```python
from build123d import *

# Parameters (mm, degrees)
CROQUIS4_R                = 1.5
SALIENTE_EXTRUIR1_DEPTH   = 5
SALIENTE_EXTRUIR1_2_DEPTH = 5
SALIENTE_EXTRUIR1_3_DEPTH = 5
SALIENTE_EXTRUIR2_START   = -3
CROQUIS5_R                = 1.5
SALIENTE_EXTRUIR2_DEPTH   = 3


with BuildPart() as part:
    # Croquis4 → Saliente-Extruir1 (new body)
    with BuildSketch(Plane.XY):
        with BuildLine():
            Line((31.332082611, 76.5), (31.332082611, 73.5))
            ThreePointArc((31.332082611, 73.5), (17.593960897, 62.317888205), (18.123970441, 44.612106598))
            Line((18.123970441, 44.612106598), (33.120139436, 16.408414688))
            ThreePointArc((33.120139436, 16.408414688), (31.879711346, 12.351157221), (27.822453879, 13.591585312))
            Line((27.822453879, 13.591585312), (17.849832742, 32.347357814))
            ThreePointArc((17.849832742, 32.347357814), (16.010285152, 34.285836504), (13.435094777, 35))
            Line((13.435094777, 35), (8.180668456, 35))
            ThreePointArc((8.180668456, 35), (4.835015424, 33.715724127), (3.208058979, 30.522642316))
            Line((3.208058979, 30.522642316), (1.105974274, 10.522642316))
            Line((1.105974274, 10.522642316), (-1.894025726, 10.522642316))
            Line((-1.894025726, 10.522642316), (-1.894025726, 27.20144431))
            ThreePointArc((-1.894025726, 27.20144431), (-0.837875871, 33.61475404), (2.219028442, 39.350722155))
            ThreePointArc((2.219028442, 39.350722155), (5.275932756, 45.086690271), (6.332082611, 51.5))
            ThreePointArc((6.332082611, 51.5), (13.654413081, 69.17766953), (31.332082611, 76.5))
        make_face()
        with Locations((11.817302712, 43.692896695)):
            Circle(CROQUIS4_R, mode=Mode.SUBTRACT)
    extrude(amount=SALIENTE_EXTRUIR1_DEPTH)



with BuildPart() as body_2:
    # Croquis4 → Saliente-Extruir1 2 (new body)
    with BuildSketch(Plane.XY):
        with BuildLine():
            Line((7.851255977, 26.865849621), (7.341304596, 22.013986331))
            ThreePointArc((7.341304596, 22.013986331), (7.719149951, 20.309636075), (9.046614258, 19.17587445))
            Line((9.046614258, 19.17587445), (17.853810231, 15.617536301))
            ThreePointArc((17.853810231, 15.617536301), (19.658030518, 16.034073375), (19.883693385, 17.871949935))
            Line((19.883693385, 17.871949935), (14.422399186, 28.14315047))
            ThreePointArc((14.422399186, 28.14315047), (10.664251127, 29.935695142), (7.851255977, 26.865849621))
        make_face()
        with Locations((11.332082611, 26.5)):
            Circle(CROQUIS4_R, mode=Mode.SUBTRACT)
    extrude(amount=SALIENTE_EXTRUIR1_2_DEPTH)


with BuildPart() as body_3:
    # Croquis4 → Saliente-Extruir1 3 (new body)
    with BuildSketch(Plane.XY):
        with BuildLine():
            Line((6.52097346, 14.209056927), (5.631578058, 5.747024927))
            Line((5.631578058, 5.747024927), (12, 5.747024927))
            Line((12, 5.747024927), (12, 14.747024927))
            Line((12, 14.747024927), (9.259230437, 15.854367709))
            ThreePointArc((9.259230437, 15.854367709), (7.479941101, 15.714334601), (6.52097346, 14.209056927))
        make_face()
    extrude(amount=SALIENTE_EXTRUIR1_3_DEPTH)


with BuildPart() as part_1:
    add(part.part)

    add(body_2.part)  # Saliente-Extruir2 merges body 2

    add(body_3.part)  # Saliente-Extruir2 merges body 3
    # Croquis5 → Saliente-Extruir2 (add)
    with BuildSketch(Plane.XY.offset(SALIENTE_EXTRUIR2_START)):
        with BuildLine():
            Line((12, 5.747024927), (31.411206338, 12.151040577))
            ThreePointArc((31.411206338, 12.151040577), (33.255375434, 13.882455653), (33.120139436, 16.408414688))
            Line((33.120139436, 16.408414688), (17.114988269, 46.509726071))
            ThreePointArc((17.114988269, 46.509726071), (11.909057427, 49.692195076), (6.608237363, 46.670418851))
            Line((6.608237363, 46.670418851), (3.695633773, 41.574926144))
            ThreePointArc((3.695633773, 41.574926144), (2.994485151, 40.43815831), (2.219028442, 39.350722155))
            ThreePointArc((2.219028442, 39.350722155), (-0.837875871, 33.61475404), (-1.894025726, 27.20144431))
            Line((-1.894025726, 27.20144431), (-1.894025726, 10.522642316))
            Line((-1.894025726, 10.522642316), (1.105974274, 10.522642316))
            Line((1.105974274, 10.522642316), (5.631578058, 5.747024927))
            Line((5.631578058, 5.747024927), (12, 5.747024927))
        make_face()
        with Locations((11.332082611, 26.5)):
            Circle(CROQUIS5_R, mode=Mode.SUBTRACT)
        with Locations((11.817302712, 43.692896695)):
            Circle(CROQUIS5_R, mode=Mode.SUBTRACT)
    extrude(amount=SALIENTE_EXTRUIR2_DEPTH)


solid = part_1.part
```
The listing builds one solid part. Answer for the finished solid, in the listing's coordinates (mm). A direction names the side the tool comes from. Give positions to 0.01 mm unless a question says otherwise; leave off trailing zeros. Order: outer loops, then holes, each group sorted by start corner. A loop starts at its lowest first (then second) coordinate and runs counter-clockwise, first axis right, second up.
Item 1: The part is cut by section B-B, the plane y = 21. Give the vertices of the cut face in (x, z).
From the geometry:
outline: (-1.89, -3) - (30.68, -3) - (30.68, 5) - (23.88, 5) - (23.88, 0) - (18.22, 0) - (18.22, 5) - (7.42, 5) - (7.42, 0) - (2.21, 0) - (2.21, 5) - (-1.89, 5) - close
Item 2: The part is cut by section A-A, the plane z = 1.5. Give the vertices of the cut face in (x, y), and give its area (3 significant figures).
From the geometry:
outline: (-1.89, 10.52) - (1.11, 10.52) - (3.21, 30.52) arc R5 cw to (8.18, 35) - (13.44, 35) arc R5 cw to (17.85, 32.35) - (27.82, 13.59) arc R3 ccw to (33.12, 16.41) - (18.12, 44.61) arc R20 cw to (31.33, 73.5) - (31.33, 76.5) arc R25 ccw to (6.33, 51.5) arc R20 cw to (2.22, 39.35) arc R20 ccw to (-1.89, 27.2) - close; (5.63, 5.75) - (12, 5.75) - (12, 14.75) - (9.26, 15.85) arc R2 ccw to (6.52, 14.21) - close; (7.34, 22.01) arc R2.75 ccw to (9.05, 19.18) - (17.85, 15.62) arc R1.61 ccw to (19.88, 17.87) - (14.42, 28.14) arc R3.5 ccw to (7.85, 26.87) - close; hole circle Ø3 at (11.33, 26.5); hole circle Ø3 at (11.82, 43.69)
area: 888 mm2
Item 3: Given pin 1 Ø1.5 at (x, z) = (14, 3) entering from +Y; pin 2 Ø1 at (x, z) = (20.5, 1.5) entering from +Y; pin 3 Ø2.5 at (y, z) = (12.5, 2.5) entering from +X, each flat-ended and moving along its own axis, determine where each tip first touches the part or whether it passes through.
From the geometry:
pin 1: stops at y = 70.21
pin 2: stops at y = 74.27
pin 3: stops at x = 33.2
Item 4: Which of the six approach directions +Z, -Z, +X, -X, +Y, -Y give full straight-line access (tool end or side, diameter ignored) to faces 1 (the face through (12, 10, 2)), 2 (the face through (31.332, 75, 2)), 3 (the face through (6.083, 10.037, 2.465))?
From the geometry:
face 1: +Z, -Y
face 2: +Z, -Z, +X, +Y
face 3: +Z
Item 5: Find the intervals of material crossed by probe 1 along Y at (x, z) = (18, 1.25); probe 2 along Y at (x, z) = (9.5, 1.25); probe 3 along Y at (x, z) = (10, 4.25), in increasing order.
From the geometry:
probe 1: y = 15.57 to 21.41, 32.06 to 44.85, 63.15 to 72.65
probe 2: y = 5.75 to 15.76, 18.99 to 29.48, 35 to 63.68
probe 3: y = 5.75 to 15.56, 18.79 to 25.81, 27.19 to 29.74, 35 to 64.54
Item 6: The part is cut by section C-C, the plane y = 63. Give the vertices of the cut face in (x, z).
From the geometry:
outline: (9.13, 0) - (17.92, 0) - (17.92, 5) - (9.13, 5) - close
